```python
from build123d import *

# Parameters (mm, degrees)
BOSS_EXTRUDE1_DEPTH         = 317.499999
BOSS_EXTRUDE1_DEPTH_BACK    = 317.499999
SKETCH3_W                   = 38.1
SKETCH3_H                   = 25.4
SKETCH3_W_2                 = 31.75
SKETCH3_H_2                 = 19.05
F_10_CLEARANCE_HOLE2_D      = 4.9784
F_10_CLEARANCE_HOLE4_D      = 4.9784
F_10_CLEARANCE_HOLE3_D      = 4.9784
F_10_CLEARANCE_HOLE5_D      = 4.9784
F_10_CLEARANCE_HOLE6_D      = 4.9784
F_1_4_0_25_DIAMETER_HOLE1_D = 6.35


with BuildPart() as part:
    # Sketch3 → Boss-Extrude1 (new, two sides: drawn at the far end of the back side and taken through both)
    with BuildSketch(Plane.XY.offset(-BOSS_EXTRUDE1_DEPTH_BACK)):
        Rectangle(SKETCH3_W, SKETCH3_H)
        Rectangle(SKETCH3_W_2, SKETCH3_H_2, mode=Mode.SUBTRACT)
    extrude(amount=BOSS_EXTRUDE1_DEPTH + BOSS_EXTRUDE1_DEPTH_BACK)

    # #10 Clearance Hole2 (through all)
    with Locations(Plane.ZY.offset(19.05)):
        with Locations((-304.800000508, 0), (-279.400000508, 0), (279.399999492, 0), (304.799999492, 0)):
            Hole(F_10_CLEARANCE_HOLE2_D / 2)

    # #10 Clearance Hole4 (through all)
    with Locations(Plane(origin=(19.05, 0, 0), x_dir=(0, 0, -1), z_dir=(1, 0, 0))):
        with Locations((-252.857000506, 8e-09), (-227.457000506, 1.1e-08), (-124.587000507, 1.943404818), (-99.187000507, 1.943404821)):
            Hole(F_10_CLEARANCE_HOLE4_D / 2)

    # #10 Clearance Hole3 (through all)
    with Locations(Plane.ZY.offset(19.05)):
        with Locations((-50.8, 0), (50.8, 0)):
            Hole(F_10_CLEARANCE_HOLE3_D / 2)

    # #10 Clearance Hole5 (through all)
    with Locations(Plane(origin=(19.05, 0, 0), x_dir=(0, 0, -1), z_dir=(1, 0, 0))):
        with Locations((82.55, 0)):
            Hole(F_10_CLEARANCE_HOLE5_D / 2)

    # #10 Clearance Hole6 (through all)
    with Locations(Plane(origin=(0, -12.7, 0), x_dir=(-1, 0, 0), z_dir=(0, -1, 0))):
        with Locations((-12.466755932, -76.754257499), (-12.466755932, 88.899999492)):
            Hole(F_10_CLEARANCE_HOLE6_D / 2)

    # 1/4 (0.25) Diameter Hole1 (through all)
    with Locations(Plane.ZY.offset(19.05)):
        with Locations((69.85, 4.2), (-64.797229307, 4.2)):
            Hole(F_1_4_0_25_DIAMETER_HOLE1_D / 2)


solid = part.part
```
The model under review builds one solid part; all positions refer to its coordinate system, in mm. A direction names the side the tool comes from. Round coordinates to 2 decimals unless told otherwise and drop trailing zeros. Write each loop counter-clockwise with the first axis right and the second up, starting at its lowest first coordinate (ties: lowest second). Pieces come first, ordered by that corner, then holes. Notation, with made-up numbers: (36.5, 25.25) - (71.5, 25.25) arc R23 ccw to (71.5, 40.25) - close; hole circle Ø11 at (55, 82.5). An arc over 180 degrees is marked (long way). One line per question, with ' | ' between items.
Item 1: To check wall thickness, follow probe 1 along X at (y, z) = (3.5, -14.5) (3 decimals); probe 2 along Y at (x, z) = (7.5, -93) (3 decimals). State the ranges of each line that lie inside material, in increasing order.
Resolved:
probe 1: x = -19.05 to -15.875, 15.875 to 19.05 | probe 2: y = -12.7 to -9.525, 9.525 to 12.7
Item 2: The part is to be moulded in two halves that separate along X. For faces 3 (the face through (-19.05, 0, -4)), 4 (the face through (0, 12.7, -4)), 5 (the face through (15.875, 0, -4)), say which applies: pulls with the +X half, pulls with the -X half, needs draft (parallel to the pull), parting line crosses it, or undercut.
Resolved:
face 3: pulls with the -X half | face 4: needs draft | face 5: undercut
Item 3: Add section B-B, the plane z = -154.5. Give the boundary of the cut face in (x, y) (3 decimals).
Resolved:
outline: (-19.05, -12.7) - (19.05, -12.7) - (19.05, 12.7) - (-19.05, 12.7) - close; hole (-15.875, -9.525) - (15.875, -9.525) - (15.875, 9.525) - (-15.875, 9.525) - close
Item 4: Add section A-A, the plane x = -0.5. Give the boundary of the cut face in (y, z) (3 decimals), then the cut area to 3 significant figures.
Resolved:
outline: (-12.7, -317.5) - (-9.525, -317.5) - (-9.525, 317.5) - (-12.7, 317.5) - close; (9.525, -317.5) - (12.7, -317.5) - (12.7, 317.5) - (9.525, 317.5) - close | area: 4,030 mm2
Item 5: For faces 1 (the face through (0, -9.525, -4)), 2 (the face through (19.05, 0, -4)), list the 3-axis set-ups (+Z, -Z, +X, -X, +Y, -Y) from which the entire face can be reached by the end or side of a thin tool; tool diameter is ignored.
Resolved:
face 1: +Z, -Z | face 2: +Z, -Z, +X, +Y, -Y
Item 6: For P1, Ø8, axis at x = 8, y = -9, coming from the -Z side, flat-tipped, find the tip position at first contact; note if it passes through.
Resolved:
P1: stops at z = -317.5
